Design review of the part shown in the three views and the two pictorial views. Dimensions are in mm from the part's minimum x, y and z. A direction names the side the tool comes from. Give positions to 0.01 mm unless a question says otherwise; leave off trailing zeros. Loops run counter-clockwise (first coordinate to the right, second up) from the corner with the lowest first, then second, coordinate; pieces in that order, holes last. Notation, with made-up numbers: (-10, -5) - (32, -5) arc R31 ccw to (32, 20) - close; hole circle Ø7 at (54.5, 79.5). An arc over 180 degrees is marked (long way). Answer as a JSON object with one key per item and string values.
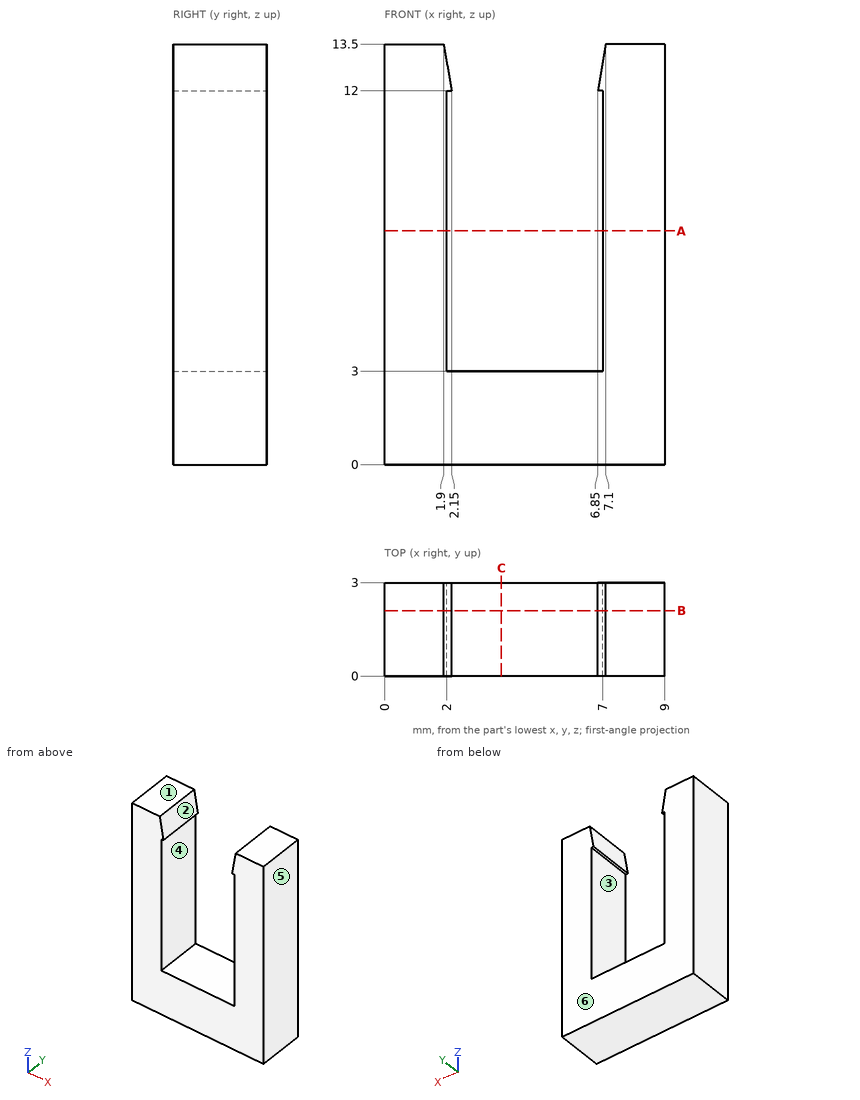
Q1. Consider section C-C, the plane x = 3.75. State the section outline as (y, z) points, plus the area to 3 significant figures.
Results:
{"outline": "(0, 0) - (3, 0) - (3, 3) - (0, 3) - close", "area": "9.00 mm^2"}
Q2. Consider section A-A, the plane z = 7.5. State the section outline as (x, y) points.
Results:
{"outline": "(0, 0) - (2, 0) - (2, 3) - (0, 3) - close; (7, 0) - (9, 0) - (9, 3) - (7, 3) - close"}
Q3. To check wall thickness, follow probe 1 along X at (y, z) = (1, 5); probe 2 along Z at (x, y) = (4, 1). State the ranges of each line that lie inside material, in increasing order. Write a range as [from, to].
Results:
{"probe 1": "x = [0, 2], [7, 9]", "probe 2": "z = [0, 3]"}
Q4. Consider section B-B, the plane y = 2.1. State the section outline as (x, z) points, plus the area to 3 significant figures.
Results:
{"outline": "(0, 0) - (9, 0) - (9, 13.5) - (7.1, 13.5) - (6.85, 12) - (7, 12) - (7, 3) - (2, 3) - (2, 12) - (2.15, 12) - (1.9, 13.5) - (0, 13.5) - close", "area": "69.1 mm^2"}
Q5. The part is to be moulded in two halves that separate along X. For the marked faces 3, 4, 5 and 6, say which applies: +X half, -X half, draft (parallel to the pull), parting line (faces both ways), or undercut.
Results:
{"face 3": "undercut", "face 4": "undercut", "face 5": "+X half", "face 6": "draft"}
Q6. For the marked faces 1 and 2, list the 3-axis set-ups (+Z, -Z, +X, -X, +Y, -Y) from which the entire face can be reached by the end or side of a thin tool; tool diameter is ignored.
Results:
{"face 1": "+Z, +X, -X, +Y, -Y", "face 2": "+Z, +Y, -Y"}
